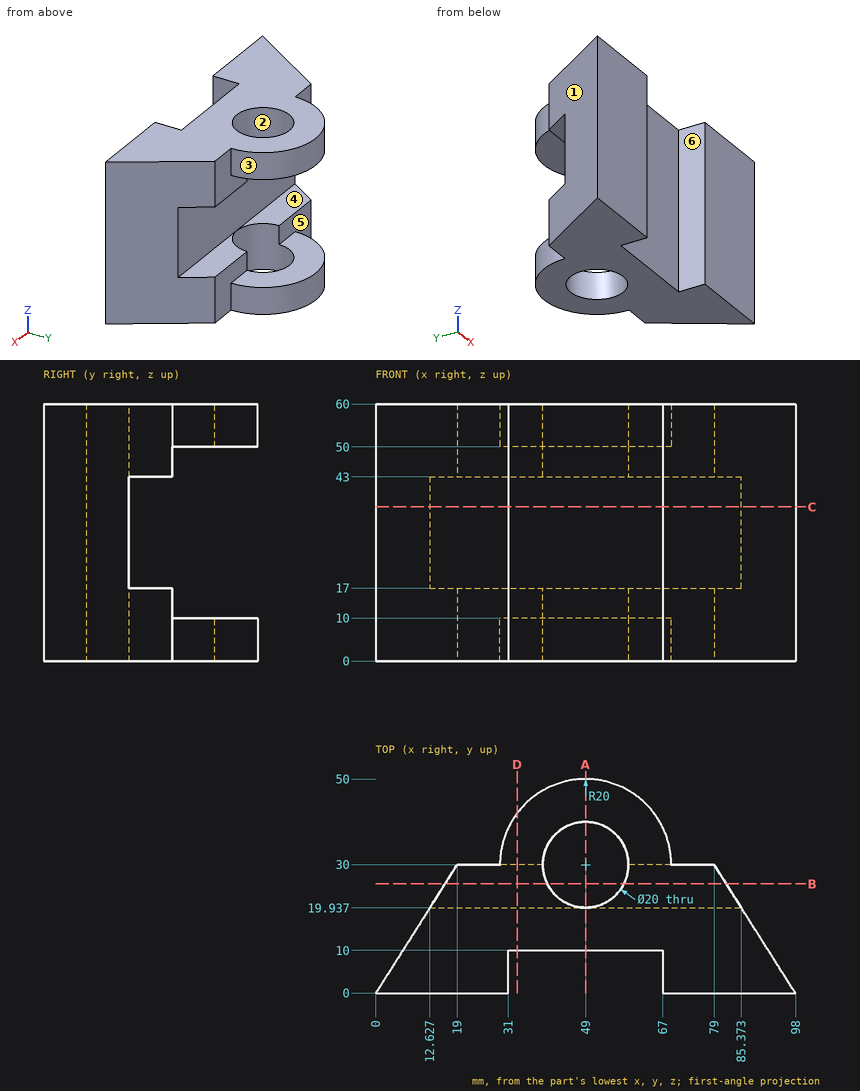
The figure shows three views and two pictorial views of one solid part (mm, origin at its lowest corner). Answer the questions. A direction names the side the tool comes from. Round coordinates to 2 decimals unless told otherwise and drop trailing zeros. Write each loop counter-clockwise with the first axis right and the second up, starting at its lowest first coordinate (ties: lowest second). Pieces come first, ordered by that corner, then holes. Notation, with made-up numbers: (-6, 50) - (17, 50) arc R22 cw to (17, 60) - close; hole circle Ø11 at (30, 41). An arc over 180 degrees is marked (long way). Answer in a Markdown table with one row per item. Add a question column.
1. Find the intervals of material crossed by line 1 along Z through (x, y) = (48, 45); line 2 along Y through (x, z) = (49, 8.25); line 3 along Y through (x, z) = (22.5, 32.5), in increasing order. Write a range as from..to.
2. A cutting plane is placed at D-D, the plane x = 33. Determine the outline of the cut face in (y, z), and give its area (3 significant figures).
3. The mould has two halves that part along X. Classify the marked faces 1, 2 and 3: +X half, -X half, draft (parallel to the pull), parting line (faces both ways), or undercut.
4. A cutting plane is placed at A-A, the plane x = 49. Determine the outline of the cut face in (y, z), and give its area (3 significant figures).
5. A cutting plane is placed at C-C, the plane z = 36. Determine the outline of the cut face in (x, y), and give its area (3 significant figures).
6. Given pin 1 (4 mm diameter, centred on y = 16, z = 50.5, fed in from +X); pin 2 (8.5 mm diameter, centred on x = 68.5, z = 52, fed in from +Y); pin 3 (10 mm diameter, centred on x = 77.5, z = 18, fed in from +Y); pin 4 (16 mm diameter, centred on x = 49, y = 30, fed in from +Z), each flat-ended and moving along its own axis, determine where each tip first touches the part or whether it passes through.
7. A cutting plane is placed at B-B, the plane y = 25.5. Determine the outline of the cut face in (x, z).
8. For the marked faces 4, 5 and 6, determine the directions among +Z, -Z, +X, -X, +Y, -Y from which every point of the face is accessible in a straight line to the end or side of a thin tool.
Worked out:
| question | item | result |
|---|---|---|
| 1 | line 1 | 0..10, 50..60 |
| 1 | line 2 | 10..20, 40..50 |
| 1 | line 3 | 0..19.94 |
| 2 | outline | (10, 0) - (42, 0) - (42, 10) - (30, 10) - (30, 17) - (19.94, 17) - (19.94, 43) - (30, 43) - (30, 50) - (42, 50) - (42, 60) - (10, 60) - close |
| 2 | area | 1,180 mm^2 |
| 3 | face 1 | -X half |
| 3 | face 2 | undercut |
| 3 | face 3 | parting line |
| 4 | outline | (10, 0) - (20, 0) - (20, 17) - (19.94, 17) - (19.94, 43) - (20, 43) - (20, 60) - (10, 60) - close; (40, 0) - (50, 0) - (50, 10) - (40, 10) - close; (40, 50) - (50, 50) - (50, 60) - (40, 60) - close |
| 4 | area | 798 mm^2 |
| 5 | outline | (0, 0) - (31, 0) - (31, 10) - (67, 10) - (67, 0) - (98, 0) - (85.37, 19.94) - (12.63, 19.94) - close |
| 5 | area | 1,340 mm^2 |
| 6 | pin 1 | x = 89.13 |
| 6 | pin 2 | y = 42.94 |
| 6 | pin 3 | y = 30 |
| 6 | pin 4 | through |
| 7 | outline | (16.15, 0) - (40.07, 0) - (40.07, 17) - (16.15, 17) - close; (16.15, 43) - (40.07, 43) - (40.07, 60) - (16.15, 60) - close; (57.93, 0) - (81.85, 0) - (81.85, 17) - (57.93, 17) - close; (57.93, 43) - (81.85, 43) - (81.85, 60) - (57.93, 60) - close |
| 8 | face 4 | +X, -X, +Y |
| 8 | face 5 | -X, +Y |
| 8 | face 6 | +Z, -Z, -Y |
